Input: part model. Units: mm. Frame: model coordinates. A direction names the side the tool comes from. Coordinates: 2 decimals unless noted, no trailing zeros. Loops run counter-clockwise (first coordinate to the right, second up) from the corner with the lowest first, then second, coordinate; pieces in that order, holes last.
(1) Section B-B, the plane z = 5.08. Return loops of the section in (x, y), then the cut area to 3 significant figures.
(2) Section C-C, the plane y = 3.5. Return loops of the section in (x, z) (3 decimals).
(3) Contact query for flat-ended pins moving along their axis: P1, Ø7, axis at x = 52, z = -13, coming from the +Y side; P2, Ø2.5, axis at x = 4, y = 10.5, coming from the +Z side; P3, Ø5, axis at y = 8, z = -11, coming from the -X side; P4, Ø4, axis at x = 51.5, y = 10.5, coming from the -Z side. Output: stop coordinate, or through.
(4) Line query: L1, parallel to X at y = 2.55, z = -12.7; L2, parallel to Z at x = 49, y = 7; L3, parallel to X at y = 5.5, z = -5.25. Output: solid intervals per line, ascending.
(5) Section A-A, the plane z = 1.75. Return loops of the section in (x, y), then the cut area to 3 significant figures.
(6) Set-up query: faces 4 (the face through (49.53, 3, 5)), 5 (the face through (6.35, 3, -12)), 6 (the face through (5, 5.08, -11)), 7 (the face through (48.26, 7, -1)). Return all of +Z, -Z, +X, -X, +Y, -Y with unobstructed straight access to the full face (end or side cutting, diameter ignored); none if empty.
(7) Section D-D, the plane z = -1.5. Return loops of the section in (x, y), then the cut area to 3 significant figures.
(8) Mould query, pull axis Z, two halves, no side actions, for faces 1 (the face through (53, 3, 8.89)), 2 (the face through (55.88, 4, -4)), 3 (the face through (2, 7, -5.08)). Classes: released by +Z, released by -Z, zero draft, split by the parting line, or undercut.
```python
from build123d import *

# Parameters (mm, degrees)
SKETCH1_R           = 2.032
BOSS_EXTRUDE1_DEPTH = 7.62
SKETCH3_W           = 2.54
SKETCH3_H           = 7.62
CUT_EXTRUDE1_DEPTH  = 55.88
SKETCH5_W           = 6.35
SKETCH5_H           = 8.89
SKETCH5_R           = 1.778
BOSS_EXTRUDE2_DEPTH = 5.08
FILLET2_R           = 4.064


with BuildPart() as part:
    # Sketch1 → Boss-Extrude1 (new body)
    with BuildSketch(Plane.XY):
        Polygon((0, 0), (0, 12.7), (7.62, 12.7), (7.62, 5.08), (48.26, 5.08), (48.26, 12.7), (55.88, 12.7), (55.88, 0), align=None)
        with Locations((3.81, 8.89)):
            Circle(SKETCH1_R, mode=Mode.SUBTRACT)
        with Locations((52.07, 8.89)):
            Circle(SKETCH1_R, mode=Mode.SUBTRACT)
    extrude(amount=-BOSS_EXTRUDE1_DEPTH)

    # Sketch3 → Cut-Extrude1 (cut)
    with BuildSketch(Plane(origin=(55.88, 0, 0), x_dir=(0, 0, -1), z_dir=(1, 0, 0))):
        with Locations((3.81, 8.89)):
            Rectangle(SKETCH3_W, SKETCH3_H)
    extrude(amount=-CUT_EXTRUDE1_DEPTH, mode=Mode.SUBTRACT)

    # Sketch5 → Boss-Extrude2 (add)
    # profile 1 of 4: a face of its own
    with BuildSketch(Plane(origin=(0, 0, 0), x_dir=(1, 0, 0), z_dir=(0, 1, 0))):
        with Locations((52.705, 12.065)):
            Rectangle(SKETCH5_W, SKETCH5_H)
        with Locations(Location((52.705, 12.7, 0), (0, 0, 270))):
            Circle(SKETCH5_R, mode=Mode.SUBTRACT)
    # profile 2 of 4: a face of its own
    with BuildSketch(Plane(origin=(0, 0, 0), x_dir=(1, 0, 0), z_dir=(0, 1, 0))):
        with Locations((52.705, -4.445)):
            Rectangle(SKETCH5_W, SKETCH5_H)
        with Locations(Location((52.705, -5.08, 0), (0, 0, 270))):
            Circle(SKETCH5_R, mode=Mode.SUBTRACT)
    # profile 3 of 4: a face of its own
    with BuildSketch(Plane(origin=(0, 0, 0), x_dir=(1, 0, 0), z_dir=(0, 1, 0))):
        with Locations((3.175, -4.445)):
            Rectangle(SKETCH5_W, SKETCH5_H)
        with Locations(Location((3.175, -5.08, 0), (0, 0, 270))):
            Circle(SKETCH5_R, mode=Mode.SUBTRACT)
    # profile 4 of 4: a face of its own
    with BuildSketch(Plane(origin=(0, 0, 0), x_dir=(1, 0, 0), z_dir=(0, 1, 0))):
        with Locations((3.175, 12.065)):
            Rectangle(SKETCH5_W, SKETCH5_H)
        with Locations(Location((3.175, 12.7, 0), (0, 0, 270))):
            Circle(SKETCH5_R, mode=Mode.SUBTRACT)
    extrude(amount=BOSS_EXTRUDE2_DEPTH)

    # Fillet2
    fillet2_edges = [part.edges().sort_by_distance(p)[0] for p in [
        (7.62, 12.7, -6.35),
        (48.26, 12.7, -6.35),
        (48.26, 12.7, -1.27),
        (7.62, 12.7, -1.27),
    ]]
    fillet(fillet2_edges, radius=FILLET2_R)


solid = part.part
```
Report:
1. outline: (0, 0) - (1.4, 0) - (1.4, 5.08) - (0, 5.08) - close; (4.95, 0) - (6.35, 0) - (6.35, 5.08) - (4.95, 5.08) - close; (49.53, 0) - (50.93, 0) - (50.93, 5.08) - (49.53, 5.08) - close; (54.48, 0) - (55.88, 0) - (55.88, 5.08) - (54.48, 5.08) - close
1. area: 28.4 mm2
2. outline: (0, -16.51) - (6.35, -16.51) - (6.35, -7.62) - (49.53, -7.62) - (49.53, -16.51) - (55.88, -16.51) - (55.88, 8.89) - (49.53, 8.89) - (49.53, 0) - (6.35, 0) - (6.35, 8.89) - (0, 8.89) - close; hole circle Ø3.556 at (3.175, -12.7); hole circle Ø3.556 at (3.175, 5.08); hole circle Ø3.556 at (52.705, -12.7); hole circle Ø3.556 at (52.705, 5.08)
3. P1: stops at y = 5.08
3. P2: stops at z = 0
3. P3: passes through
3. P4: stops at z = -7.62
4. L1: x = 0 to 1.4, 4.95 to 6.35, 49.53 to 50.93, 54.48 to 55.88
4. L2: z = -7.62 to -5.08, -2.54 to 0
4. L3: x = 0 to 7.62, 48.26 to 55.88
5. outline: (0, 0) - (6.35, 0) - (6.35, 5.08) - (0, 5.08) - close; (49.53, 0) - (55.88, 0) - (55.88, 5.08) - (49.53, 5.08) - close
5. area: 64.5 mm2
6. face 4: +Z, +Y, -Y
6. face 5: -Z, +Y, -Y
6. face 6: -Z, +X, -X, +Y
6. face 7: +Z, -Z, +Y
7. outline: (0, 0) - (55.88, 0) - (55.88, 12.7) - (52.32, 12.7) arc R4.06 ccw to (48.26, 8.64) - (48.26, 5.08) - (7.62, 5.08) - (7.62, 8.64) arc R4.06 ccw to (3.56, 12.7) - (0, 12.7) - close; hole circle Ø4.06 at (3.81, 8.89); hole circle Ø4.06 at (52.07, 8.89)
7. area: 367 mm2
8. face 1: released by +Z
8. face 2: zero draft
8. face 3: undercut
